Geometry: final body of the model. Coordinates: model frame, mm. A direction names the side the tool comes from. Coordinates: 2 decimals unless noted, no trailing zeros. Order: outer loops, then holes, each group sorted by start corner. A loop starts at its lowest first (then second) coordinate and runs counter-clockwise, first axis right, second up. Notation, with made-up numbers: M 28.25,-28.5 L 56.25,-28.5 A26 ccw 56.25,-4.5 Z; hole C 12.5,76.25 d11. An arc over 180 degrees is marked long. Use CSV: the item, a comma, the result in double quotes. Start each with the question number.
Q1. Ray query, probe 1 along X at (y, z) = (-2.05, 0.5); probe 2 along X at (y, z) = (-0.6, -0.55); probe 3 along Z at (x, y) = (3.75, -0.05). Return the intervals inside material, ascending.
Q2. Section query B-B, the plane x = 3.25. Output: boundary loops of the cut face in (y, z), and give its area (3 significant figures).
Q3. Access query for faces 5 (the face through (-1, -0.996, 0)), 6 (the face through (-2, 1.2, 0)), 7 (the face through (0, 2, 0)). Directions: +Z, -Z, +X, -X, +Y, -Y. A direction counts if a zero-diameter tool reaches every point of the face in a straight line with its end or side. Return the directions, or none.
Q4. Section query C-C, the plane y = -2.4. Output: boundary loops of the cut face in (x, z).
Q5. First-contact query: P1, Ø0.5, axis at y = 0.5, z = 0, coming from the -X side; P2, Ø1, axis at x = 5, z = 0, coming from the -Y side. Flat tips, straight axial feed; report the tip coordinate or a pass-through.
Q6. Mould query, pull axis Z, two halves, no side actions, for faces 1 (the face through (15, 0, 0)), 2 (the face through (-0.986, -0.596, -2.685)), 3 (the face through (-1.408, 0.491, -0.867)), 4 (the face through (-1.408, -0.491, 0.867)). Classes: +Z half, -Z half, draft (parallel to the pull), parting line (faces both ways), or undercut.
Q7. Section query A-A, the plane z = 0. Output: boundary loops of the cut face in (x, y).
Autodesk Inventor part; units mm, degrees
ref_plane "YZ Plane" through (0, 0, 0) normal (1, 0, 0) x (0, 1, 0)
ref_plane "XZ Plane" through (0, 0, 0) normal (0, 1, 0) x (-1, 0, 0)
ref_plane "XY Plane" through (0, 0, 0) normal (0, 0, 1) x (1, 0, 0)
sketch "スケッチ1" plane through (0, 0, 0) normal (0, 0, 1) x (1, 0, 0)
  line L0 (0, 0) -> (15, 0)
  line L1 (15, 0) -> (15, 1.5)
  line L2 (15, 1.5) -> (0, 1.5)
  line L3 (0, 1.5) -> (0, 0)
  line L4 (0, 0) -> (0, 2.75)
  line L5 (0, 0) -> (-2, 0)
  line L6 (-2, 0) -> (0, 0)
  line L7 (-2, 0) -> (-2, 1.15)
  line L8 (0, 0) -> (-2, 0)
  line L9 (-2, 0) -> (-2, 2.75)
  line L10 (-2, 2.75) -> (0, 2.75)
  line L11 (0, 2.75) -> (0, 0)
  dimension "d0" = 1.5
  dimension "d1" = 15
  dimension "d3" = 2
  dimension "d4" = 2.75
  dimension "d5" = 1.15
revolve "回転1" add sketch "スケッチ1" angle 360 about axis through (-2, 0, 0) along (1, 0, 0)
thread "ねじ1"
sketch "スケッチ2" plane through (-2, 0, 0) normal (-1, 0, 0) x (0, 0, 1)
  line L0 (-0.575, 0.9959) -> (0.575, 0.9959)
  line L1 (0.575, 0.9959) -> (1.15, 0)
  line L2 (1.15, 0) -> (0.575, -0.9959)
  line L3 (0.575, -0.9959) -> (-0.575, -0.9959)
  line L4 (-0.575, -0.9959) -> (-1.15, 0)
  line L5 (-1.15, 0) -> (-0.575, 0.9959)
  point P0 (0, 0)
  point P1 (0, 0)
  point P2 (0, 0)
  dimension "d10" = 1.15
  dimension "d11" = 1.9919
extrude "押し出し1" cut sketch "スケッチ2" against normal blind 1.4
fillet "フィレット1" radius 0.2 6 edges at (-0.6, 0.9959, 0) (-0.6, 0.498, 0.8625) (-0.6, 0.498, -0.8625) (-0.6, -0.498, -0.8625) (-0.6, -0.9959, 0) (-0.6, -0.498, 0.8625)
fillet "フィレット2" radius 0.1 1 edges at (0, -1.5, 0)
fillet "フィレット3" radius 0.1 1 edges at (15, -1.5, 0)
properties part number "ネジキャップM3L15" material "鋼"
Responses:
1,probe 1,"x = -2 to 0"
1,probe 2,"x = -0.6 to 15"
1,probe 3,"z = -1.5 to 1.5"
2,outline,"C 0,0 d3"
2,area,"7.07 mm²"
3,face 5,"-X"
3,face 6,"+Z, -Z, -X, +Y, -Y"
3,face 7,"+X"
4,outline,"M -2,-1.34 L 0,-1.34 L 0,1.34 L -2,1.34 Z"
5,P1,"stops at x = -0.6"
5,P2,"stops at y = -1.5"
6,face 1,"draft"
6,face 2,"parting line"
6,face 3,"undercut"
6,face 4,"undercut"
7,outline,"M -2,-2.75 L 0,-2.75 L 0,-1.6 A0.1 cw 0.1,-1.5 L 14.9,-1.5 A0.1 ccw 15,-1.4 L 15,1.4 A0.1 ccw 14.9,1.5 L 0.1,1.5 A0.1 cw 0,1.6 L 0,2.75 L -2,2.75 L -2,1 L -0.8,1 A0.2 cw -0.6,0.8 L -0.6,-0.8 A0.2 cw -0.8,-1 L -2,-1 Z"
